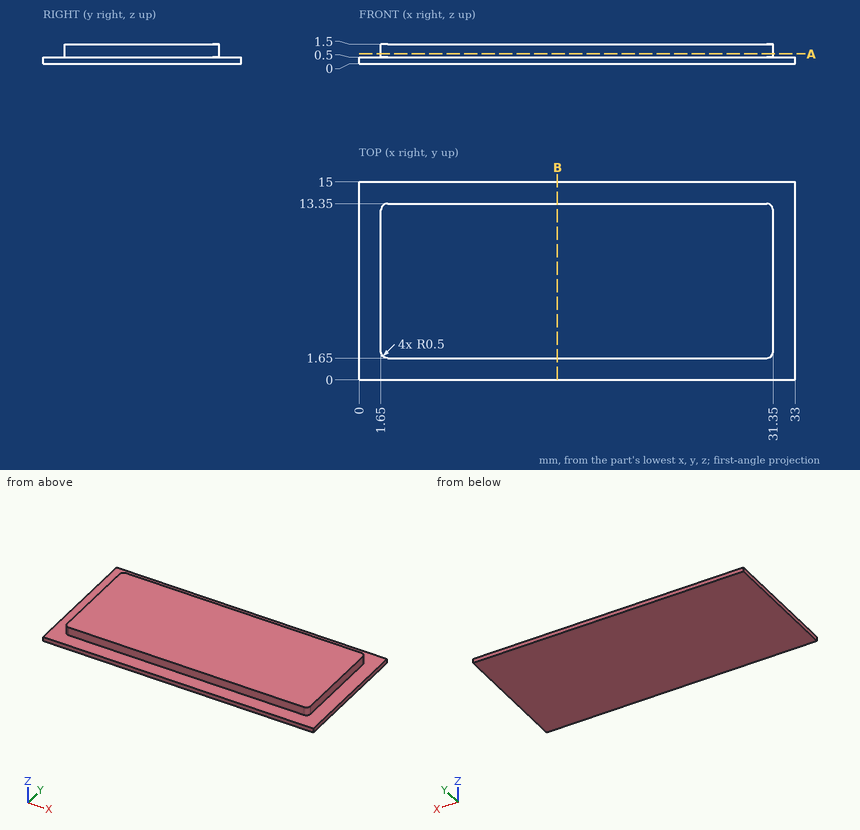
Job drawing, mm, ordinate dimensions from the low corner. One solid piece. Round coordinates to 2 decimals unless told otherwise and drop trailing zeros. Loops run counter-clockwise (first coordinate to the right, second up) from the corner with the lowest first, then second, coordinate; pieces in that order, holes last.
Item 1: Cut at B-B, the plane x = 15. Give the cut face in (y, z), then the cut area to 3 significant figures.
Item 2: Cut at A-A, the plane z = 0.75. Give the cut face in (x, y).
Item 3: Drop flat-ended pins along their axis: P1, Ø0.5, axis at y = 9, z = 1, coming from the -X side; P2, Ø0.5, axis at y = 9, z = 1, coming from the +X side; P3, Ø0.8, axis at x = 22.5, z = 1, coming from the +Y side. Give the stop position or say it passes through.
Item 4: Drill centre lines: line 1 (X direction, y = 12.25, z = 1); line 2 (Z direction, x = 8.5, y = 1.5); line 3 (Y direction, x = 5, z = 1.45). Where is each one in solid material? Low to high.
A:
1. outline: (0, 0) - (15, 0) - (15, 0.5) - (13.35, 0.5) - (13.35, 1.5) - (1.65, 1.5) - (1.65, 0.5) - (0, 0.5) - close
1. area: 19.2 mm2
2. outline: (1.65, 2.15) arc R0.5 ccw to (2.15, 1.65) - (30.85, 1.65) arc R0.5 ccw to (31.35, 2.15) - (31.35, 12.85) arc R0.5 ccw to (30.85, 13.35) - (2.15, 13.35) arc R0.5 ccw to (1.65, 12.85) - close
3. P1: stops at x = 1.65
3. P2: stops at x = 31.35
3. P3: stops at y = 13.35
4. line 1: x = 1.65 to 31.35
4. line 2: z = 0 to 0.5
4. line 3: y = 1.65 to 13.35
